```python
from build123d import *

# Parameters (mm, degrees)
BOSS_EXTRUDE1_DEPTH = 12.7
FILLET1_R           = 20


with BuildPart() as part:
    # Sketch1 → Boss-Extrude1 (new, symmetric)
    with BuildSketch(Plane.XY):
        Polygon((0, 0), (85, 0), (85, 20), (20, 85), (0, 85), align=None)
    extrude(amount=BOSS_EXTRUDE1_DEPTH, both=True)

    # Fillet1
    fillet1_edges = [part.edges().sort_by_distance(p)[0] for p in [
        (20, 85, 0),
        (85, 20, 0),
    ]]
    fillet(fillet1_edges, radius=FILLET1_R)


solid = part.part
```
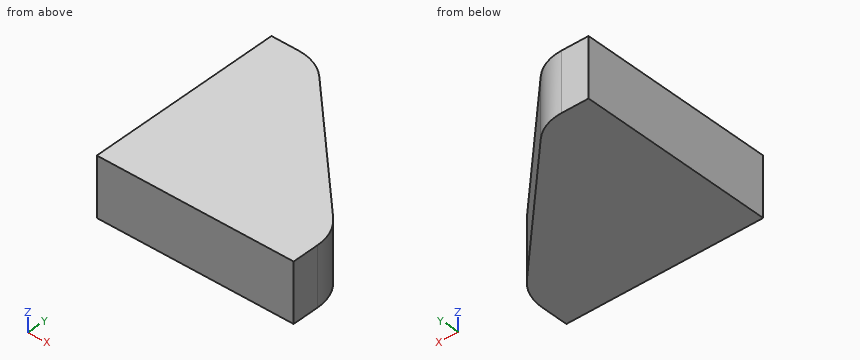
Source: CAD feature listing. Evaluate the final solid. Frame: model axes, mm. Coordinates: 2 decimals unless noted, no trailing zeros. Order: outer loops, then holes, each group sorted by start corner. A loop starts at its lowest first (then second) coordinate and runs counter-clockwise, first axis right, second up. Notation, with made-up numbers: (42.25, 48.25) - (54.25, 48.25) arc R9 cw to (54.25, 54.25) - close; hole circle Ø9 at (16.25, 58.5). An arc over 180 degrees is marked (long way). One line per item, written item: value.
1) Cut plane A-A on z = 2. Output: boundary loops of the cut face in (x, y).
Computed values:
outline: (0, 0) - (85, 0) - (85, 11.72) arc R20 ccw to (79.14, 25.86) - (25.86, 79.14) arc R20 ccw to (11.72, 85) - (0, 85) - close
2) Ray query, line 1 (Y direction, x = 12, z = -1.75); line 2 (X direction, y = 37.5, z = -2.75); line 3 (Y direction, x = 75, z = -6.5). Return the intervals inside material, ascending. Write a range as [from, to].
Computed values:
line 1: y = [0, 85]
line 2: x = [0, 67.5]
line 3: y = [0, 30]
3) Cut plane B-B on y = 74. Output: boundary loops of the cut face in (x, z), plus the area to 3 significant figures.
Computed values:
outline: (0, -12.7) - (31, -12.7) - (31, 12.7) - (0, 12.7) - close
area: 787 mm^2
4) Cut plane C-C on x = 46. Output: boundary loops of the cut face in (y, z).
Computed values:
outline: (0, -12.7) - (59, -12.7) - (59, 12.7) - (0, 12.7) - close
5) Contact query for flat-ended pins moving along their axis: pin 1 (1.5 mm diameter, centred on x = 34, y = 72.5, fed in from +Z); pin 2 (3 mm diameter, centred on y = 56.5, z = -4.5, fed in from +X); pin 3 (4 mm diameter, centred on x = 26.5, z = -7, fed in from +Y); pin 4 (2 mm diameter, centred on x = 47, z = -2, fed in from +Y). Output: stop coordinate, or through.
Computed values:
pin 1: passes through
pin 2: stops at x = 50
pin 3: stops at y = 80.38
pin 4: stops at y = 59
